Check sheet for the drawn part. Datum: minimum x, y, z corner. Units: mm. A direction names the side the tool comes from. Coordinates: 2 decimals unless noted, no trailing zeros. Loops run counter-clockwise (first coordinate to the right, second up) from the corner with the lowest first, then second, coordinate; pieces in that order, holes last. Notation, with made-up numbers: (2.25, -29) - (48.25, -29) arc R30 ccw to (48.25, 6) - close; hole circle Ø4 at (42.25, 28). An arc over 180 degrees is marked (long way). Answer as CSV lines item,"result". Start each with the question number.
1. Set-up check for the marked faces 4 and 5: record each of +Z, -Z, +X, -X, +Y, -Y from which the full face is reachable in a straight line by a thin tool's end or side.
2. Gauge pin test, flat ends, axial feed: P1, Ø2, axis at x = 635, y = 60.5, coming from the -Z side (1 decimal); P2, Ø3, axis at x = 782, y = 327, coming from the -Z side (1 decimal); P3, Ø5, axis at y = 64, z = 176, coming from the -X side (1 decimal). Record the tip position at first contact, or that the pin passes through.
3. Material ranges on line 1 (Z direction, x = 282.5, y = 23) (1 decimal); line 2 (Z direction, x = 437, y = 21) (1 decimal); line 3 (Z direction, x = 332.5, y = 389) (1 decimal), recorded low to high. Write a range as [from, to].
4. Release check for a two-part mould opening along Z. For the marked faces 1, 2 and 3 record: pulls with the +Z half, pulls with the -Z half, needs draft (parallel to the pull), parting line crosses it, or undercut.
5. Cross-section at C-C (x = 520). Enter the section's corners in (y, z) (1 decimal).
6. Cross-section at A-A (y = 33). Enter the section's corners in (x, z) (1 decimal).
7. Cross-section at D-D (x = 156). Enter the section's corners in (y, z) (1 decimal), plus the area to 3 significant figures.
8. Cross-section at B-B (z = 36). Enter the section's corners in (x, y).
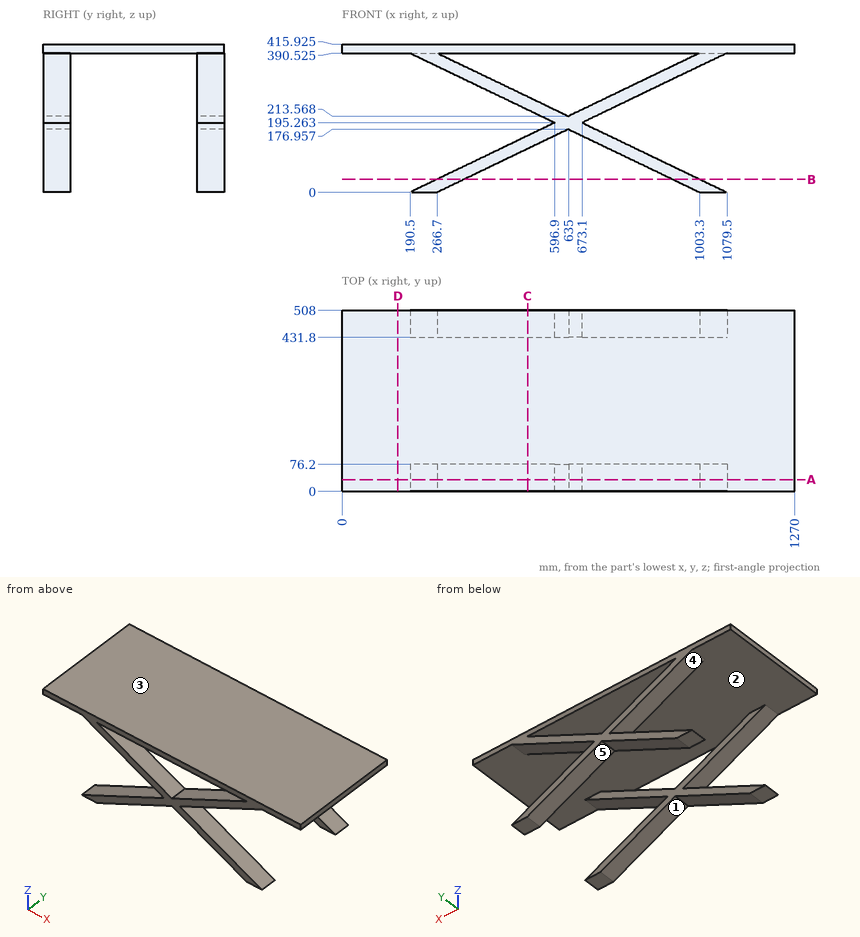
Values follow:
1,face 4,"-X, +Y, -Y"
1,face 5,"-Z, +Y, -Y"
2,P1,"stops at z = 176.5"
2,P2,"stops at z = 390.5"
2,P3,"stops at x = 551.6"
3,line 1,"z = [7.6, 44.2], [346.3, 382.9], [390.5, 415.9]"
3,line 2,"z = [81.8, 118.4], [272.1, 308.7], [390.5, 415.9]"
3,line 3,"z = [390.5, 415.9]"
4,face 1,"pulls with the -Z half"
4,face 2,"undercut"
4,face 3,"pulls with the +Z half"
5,outline,"(0, 121.7) - (76.2, 121.7) - (76.2, 158.3) - (0, 158.3) - close; (0, 232.2) - (76.2, 232.2) - (76.2, 268.8) - (0, 268.8) - close; (0, 390.5) - (508, 390.5) - (508, 415.9) - (0, 415.9) - close; (431.8, 121.7) - (508, 121.7) - (508, 158.3) - (431.8, 158.3) - close; (431.8, 232.2) - (508, 232.2) - (508, 268.8) - (431.8, 268.8) - close"
6,outline,"(0, 390.5) - (190.5, 390.5) - (596.9, 195.3) - (190.5, 0) - (266.7, 0) - (635, 177) - (1003.3, 0) - (1079.5, 0) - (673.1, 195.3) - (1079.5, 390.5) - (1270, 390.5) - (1270, 415.9) - (0, 415.9) - close; hole (266.7, 390.5) - (635, 213.6) - (1003.3, 390.5) - close"
7,outline,"(0, 390.5) - (508, 390.5) - (508, 415.9) - (0, 415.9) - close"
7,area,"12,900 mm²"
8,outline,"(265.43, 0) - (341.63, 0) - (341.63, 76.2) - (265.43, 76.2) - close; (265.43, 431.8) - (341.63, 431.8) - (341.63, 508) - (265.43, 508) - close; (928.37, 0) - (1004.57, 0) - (1004.57, 76.2) - (928.37, 76.2) - close; (928.37, 431.8) - (1004.57, 431.8) - (1004.57, 508) - (928.37, 508) - close"
